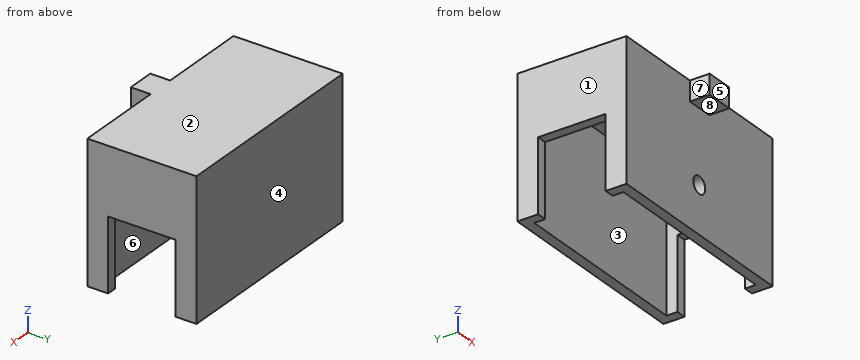
```python
from build123d import *

# Parameters (mm, degrees)
SKETCH_W        = 42
SKETCH_H        = 22
PAD_DEPTH       = 28
SKETCH001_W     = 38
SKETCH001_H     = 18
POCKET_DEPTH    = 26
SKETCH002_W     = 5.6
SKETCH002_H     = 4
PAD001_DEPTH    = 4
SKETCH003_W     = 13.6
SKETCH003_H     = 14.6
POCKET001_DEPTH = 45
SKETCH004_R     = 1.7
POCKET002_DEPTH = 5


with BuildPart() as part:
    # Sketch → Pad (new body)
    with BuildSketch(Plane.XY):
        Rectangle(SKETCH_W, SKETCH_H)
    extrude(amount=PAD_DEPTH)

    # Sketch001 (on Face5 of Pad) → Pocket (cut)
    with BuildSketch(Plane(origin=(0, 0, 0), x_dir=(1, 0, 0), z_dir=(0, 0, -1))):
        Rectangle(SKETCH001_W, SKETCH001_H)
    extrude(amount=-POCKET_DEPTH, mode=Mode.SUBTRACT)

    # Sketch002 (on Face6 of Pocket) → Pad001 (join)
    with BuildSketch(Plane.XZ.offset(11)):
        with Locations((0, 26)):
            Rectangle(SKETCH002_W, SKETCH002_H)
    extrude(amount=PAD001_DEPTH)

    # Sketch003 (on Face2 of Pad001) → Pocket001 (cut)
    with BuildSketch(Plane(origin=(-21, 0, 0), x_dir=(0, -1, 0), z_dir=(-1, 0, 0))):
        with Locations((0, 7.3)):
            Rectangle(SKETCH003_W, SKETCH003_H)
    extrude(amount=-POCKET001_DEPTH, mode=Mode.SUBTRACT)

    # Sketch004 (on Face18 of Pocket001) → Pocket002 (cut)
    with BuildSketch(Plane(origin=(0, -9, 0), x_dir=(-1, 0, 0), z_dir=(0, 1, 0))):
        with Locations((0.093022, 9.434252)):
            Circle(SKETCH004_R)
    extrude(amount=-POCKET002_DEPTH, mode=Mode.SUBTRACT)


solid = part.part
```
Check sheet for the modelled part. Datum: model origin and axes. Units: mm. Face numbers are marked on the shaded views. A direction names the side the tool comes from. Round coordinates to 2 decimals unless told otherwise and drop trailing zeros. Loops run counter-clockwise (first coordinate to the right, second up) from the corner with the lowest first, then second, coordinate; pieces in that order, holes last. Notation, with made-up numbers: (20.25, 31) - (63.25, 31) arc R17 ccw to (63.25, 60) - close; hole circle Ø8 at (67.5, 11.5). An arc over 180 degrees is marked (long way). Answer as a JSON object with one key per item and string values. Group by question number.
Q1. Gauge pin test, flat ends, axial feed: P1, Ø2, axis at y = -13.5, z = 25.5, coming from the -X side; P2, Ø12, axis at x = 15.5, z = 9.5, coming from the -Y side; P3, Ø1, axis at x = 20, y = 2.5, coming from the -Z side; P4, Ø1.5, axis at y = -5, z = 8, coming from the +X side. Record the tip position at first contact, or that the pin passes through.
Q2. Sectioned sample at B-B, the plane x = 5.5. Enter the section's corners in (y, z), plus the area to 3 significant figures.
Q3. Sectioned sample at D-D, the plane y = 0.25. Enter the section's corners in (x, z).
Q4. Sectioned sample at C-C, the plane z = 19.75. Enter the section's corners in (x, y), plus the area to 3 significant figures.
Q5. Set-up check for the marked faces 4, 5, 6, 7 and 8: record each of +Z, -Z, +X, -X, +Y, -Y from which the full face is reachable in a straight line by a thin tool's end or side.
Q6. Mould release check, pull along X, two halves, no side actions. Record for the marked faces 1, 2 and 3: released by +X, released by -X, zero draft, split by the parting line, or undercut.
Q7. Sectioned sample at A-A, the plane z = 2.5. Enter the section's corners in (x, y), plus the area to 3 significant figures.
Q8. Scan lines: line 1 along Y through (x, z) = (6.5, 7); line 2 along X through (y, z) = (-5, 21.5); line 3 along Z through (x, y) = (-2, 4.25). Record each from-to range of solid material in increasing order. Write a range as [from, to].
Solution:
{
 "1": {"P1": "stops at x = -2.8", "P2": "stops at y = -11", "P3": "stops at z = 14.6", "P4": "passes through"},
 "2": {"outline": "(-11, 0) - (-9, 0) - (-9, 26) - (9, 26) - (9, 0) - (11, 0) - (11, 28) - (-11, 28) - close", "area": "148 mm²"},
 "3": {"outline": "(-21, 14.6) - (-19, 14.6) - (-19, 26) - (19, 26) - (19, 14.6) - (21, 14.6) - (21, 28) - (-21, 28) - close"},
 "4": {"outline": "(-21, -11) - (21, -11) - (21, 11) - (-21, 11) - close; hole (-19, -9) - (19, -9) - (19, 9) - (-19, 9) - close", "area": "240 mm²"},
 "5": {"face 4": "+Z, -Z, +X, -X, +Y", "face 5": "+Z, -Z, +X, -X, -Y", "face 6": "-Z", "face 7": "+Z, -Z, -X, -Y", "face 8": "-Z, +X, -X, -Y"},
 "6": {"face 1": "released by -X", "face 2": "zero draft", "face 3": "undercut"},
 "7": {"outline": "(-21, -11) - (21, -11) - (21, -6.8) - (19, -6.8) - (19, -9) - (-19, -9) - (-19, -6.8) - (-21, -6.8) - close; (-21, 6.8) - (-19, 6.8) - (-19, 9) - (19, 9) - (19, 6.8) - (21, 6.8) - (21, 11) - (-21, 11) - close", "area": "186 mm²"},
 "8": {"line 1": "y = [-11, -9], [9, 11]", "line 2": "x = [-21, -19], [19, 21]", "line 3": "z = [26, 28]"}
}
